Part model, mm, in its own coordinate system. Give positions to 0.01 mm unless a question says otherwise; leave off trailing zeros. Order: outer loops, then holes, each group sorted by start corner. A loop starts at its lowest first (then second) coordinate and runs counter-clockwise, first axis right, second up.
1. Probe line 1 (Y direction, x = -0.5, z = -1.5). List the from-to ranges inside material, lowest first.
2. Slice it at A-A on y = -0.6. List the corners of the cut face in (x, z).
3. Slice it at C-C on z = 0.75. List the corners of the cut face in (x, y), and give its area (3 significant figures).
4. Slice it at B-B on x = 1.2. List the corners of the cut face in (y, z).
5. Drop flat-ended pins along their axis: pin 1 Ø0.8 at (x, z) = (0, -4) entering from -Y; pin 2 Ø3 at (x, z) = (-2, -5) entering from +Y. Give the stop position or say it passes through.
from build123d import *

# Parameters (mm, degrees)
BOSS_EXTRUDE1_DEPTH = 0.1
SKETCH2_R           = 0.15
BOSS_EXTRUDE2_DEPTH = 1.5
SKETCH3_R           = 2.5
BOSS_EXTRUDE3_DEPTH = 0.3
SKETCH4_R           = 0.1
CUT_EXTRUDE1_DEPTH  = 2.9


with BuildPart() as part:
    # Sketch1 → Boss-Extrude1 (new body)
    with BuildSketch(Plane(origin=(0, 0, 0), x_dir=(1, 0, 0), z_dir=(0, 1, 0))):
        with BuildLine():
            Line((-0.127906747, 0.534920428), (-0.119541068, 1.873429083))
            add(Edge.make_bspline(
                [(-0.119541068, 1.873429083), (-0.641060696, 1.506237283), (-1.004261291, 2.385988304), (-0.624353855, 3.513359347), (-0.302826258, 4.171285989)],
                knots=[0, 0, 0, 0, 0.462172684, 0.924345367, 0.924345367, 0.924345367, 0.924345367], degree=3))
            ThreePointArc((-0.302826258, 4.171285989), (-0.152583372, 4.592680906), (-0.099769187, 5.036930007))
            Line((-0.099769187, 5.036930007), (-0.052260994, 12.638240889))
            Line((-0.052260994, 12.638240889), (0.052260994, 12.638240889))
            Line((0.052260994, 12.638240889), (0.099769187, 5.036930007))
            ThreePointArc((0.099769187, 5.036930007), (0.152583372, 4.592680906), (0.302826258, 4.171285989))
            add(Edge.make_bspline(
                [(0.119541068, 1.873429083), (0.641060696, 1.506237283), (1.004261291, 2.385988304), (0.624353855, 3.513359347), (0.302826258, 4.171285989)],
                knots=[0, 0, 0, 0, 0.462172684, 0.924345367, 0.924345367, 0.924345367, 0.924345367], degree=3))
            Line((0.119541068, 1.873429083), (0.127906747, 0.534920428))
            ThreePointArc((0.127906747, 0.534920428), (0, -0.55), (-0.127906747, 0.534920428))
        make_face()
        with BuildLine():
            add(Edge.make_bspline(
                [(0, 2.187874242), (-1.052874031, 1.436460782), (-0.435783261, 3.612960551), (0, 4.238807322)],
                knots=[0, 0, 0, 0, 1, 1, 1, 1], degree=3))
            add(Edge.make_bspline(
                [(0, 2.187874242), (1.052874031, 1.436460782), (0.435783261, 3.612960551), (0, 4.238807322)],
                knots=[0, 0, 0, 0, 1, 1, 1, 1], degree=3))
        make_face(mode=Mode.SUBTRACT)
    extrude(amount=BOSS_EXTRUDE1_DEPTH)

    # Sketch2 → Boss-Extrude2 (add)
    with BuildSketch(Plane.XZ):
        Circle(SKETCH2_R)
    extrude(amount=BOSS_EXTRUDE2_DEPTH)

    # Sketch3 → Boss-Extrude3 (add)
    with BuildSketch(Plane.XZ.offset(1.5)):
        Circle(SKETCH3_R)
    extrude(amount=BOSS_EXTRUDE3_DEPTH)

    # Sketch4 → Cut-Extrude1 (cut, through all)
    with BuildSketch(Plane(origin=(0, 0.1, 0), x_dir=(1, 0, 0), z_dir=(0, 1, 0))):
        Circle(SKETCH4_R)
    extrude(amount=-CUT_EXTRUDE1_DEPTH, mode=Mode.SUBTRACT)


solid = part.part
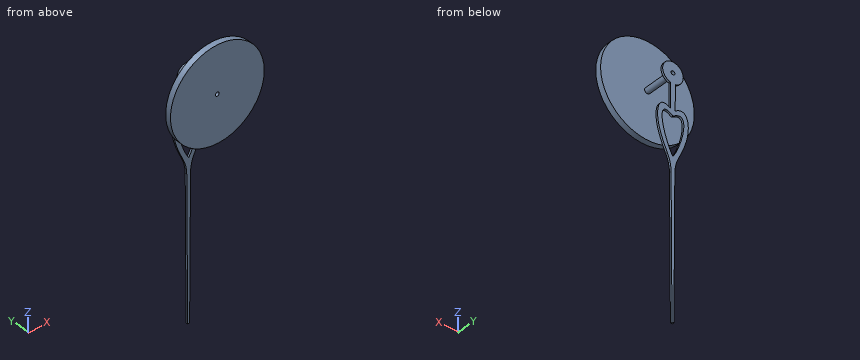
Data:
1. line 1: y = -1.8 to -1.5
2. outline: circle Ø0.3 at (0, 0); hole circle Ø0.2 at (0, 0)
3. outline: (-2.38, -1.8) - (2.38, -1.8) - (2.38, -1.5) - (-2.38, -1.5) - close
3. area: 1.43 mm2
4. outline: (-1.8, -2.19) - (-1.5, -2.19) - (-1.5, 2.19) - (-1.8, 2.19) - close
5. pin 1: stops at y = 0
5. pin 2: passes through
